For this review, take the finished solid that the model builds, in its own axes (mm). A direction names the side the tool comes from. Round coordinates to 2 decimals unless told otherwise and drop trailing zeros. Write each loop counter-clockwise with the first axis right and the second up, starting at its lowest first coordinate (ties: lowest second). Pieces come first, ordered by that corner, then holes.
from build123d import *

# Parameters (mm, degrees)
F0_R     = 12.5
F1_DEPTH = 3
F2_R     = 1
F3_DEPTH = 12.5
F4_R     = 2
F4_R_2   = 1
F5_DEPTH = 4
F7_DEPTH = 2


with BuildPart() as f1:
    # F0 (on Top) → F1 (new body, symmetric)
    with BuildSketch(Plane.XY):
        Circle(F0_R)
    extrude(amount=F1_DEPTH, both=True)

    # F2 (on Top) → F3 (cut, symmetric)
    with BuildSketch(Plane.XY):
        with Locations((0, -8)):
            Circle(F2_R)
        with Locations((-5.6568542495, -5.6568542495)):
            Circle(F2_R)
        with Locations((-8, 0)):
            Circle(F2_R)
        with Locations((-5.6568542495, 5.6568542495)):
            Circle(F2_R)
        with Locations((0, 8)):
            Circle(F2_R)
        with Locations((5.6568542495, 5.6568542495)):
            Circle(F2_R)
        with Locations((8, 0)):
            Circle(F2_R)
        with Locations((5.6568542495, -5.6568542495)):
            Circle(F2_R)
    extrude(amount=F3_DEPTH, both=True, mode=Mode.SUBTRACT)

    # F4 (on face) → F5 (cut)
    with BuildSketch(Plane.XY.offset(3)):
        with Locations((-5.6568542495, 5.6568542495)):
            Circle(F4_R)
        with Locations((-5.6568542495, 5.6568542495)):
            Circle(F4_R_2, mode=Mode.SUBTRACT)
        with Locations((-8, 0)):
            Circle(F4_R)
        with Locations((-8, 0)):
            Circle(F4_R_2, mode=Mode.SUBTRACT)
        with Locations((0, 8)):
            Circle(F4_R)
        with Locations((0, 8)):
            Circle(F4_R_2, mode=Mode.SUBTRACT)
        with Locations((8, 0)):
            Circle(F4_R)
        with Locations((8, 0)):
            Circle(F4_R_2, mode=Mode.SUBTRACT)
        with Locations((5.6568542495, 5.6568542495)):
            Circle(F4_R)
        with Locations((5.6568542495, 5.6568542495)):
            Circle(F4_R_2, mode=Mode.SUBTRACT)
        with Locations((5.6568542495, -5.6568542495)):
            Circle(F4_R)
        with Locations((5.6568542495, -5.6568542495)):
            Circle(F4_R_2, mode=Mode.SUBTRACT)
        with Locations((0, -8)):
            Circle(F4_R)
        with Locations((0, -8)):
            Circle(F4_R_2, mode=Mode.SUBTRACT)
        with Locations((-5.6568542495, -5.6568542495)):
            Circle(F4_R)
        with Locations((-5.6568542495, -5.6568542495)):
            Circle(F4_R_2, mode=Mode.SUBTRACT)
    extrude(amount=-F5_DEPTH, mode=Mode.SUBTRACT)

    # F6 (on face) → F7 (join)
    with BuildSketch(Plane.XY.offset(3)):
        Polygon((-0.2840909091, 1.25), (-1.25, 5.5), (-1.25, 1.25), align=None)
        Polygon((1.25, 5.5), (-1.25, 5.5), (-0.2840909091, 1.25), (1.25, 1.25), align=None)
        Polygon((-0.2840909091, 1.25), (-1.25, 1.25), (-1.25, -0.2840909091), (0, 0), align=None)
        Polygon((-1.25, -0.2840909091), (-1.25, 1.25), (-5.5, 1.25), (-5.5, -1.25), align=None)
        Polygon((1.25, 1.25), (-0.2840909091, 1.25), (0, 0), (1.25, 0.2840909091), align=None)
        Polygon((5.5, 1.25), (1.25, 1.25), (1.25, 0.2840909091), align=None)
        Polygon((0, 0), (-1.25, -0.2840909091), (-1.25, -1.25), (0.2840909091, -1.25), align=None)
        Polygon((-1.25, -1.25), (-1.25, -0.2840909091), (-5.5, -1.25), align=None)
        Polygon((1.25, 0.2840909091), (0, 0), (0.2840909091, -1.25), (1.25, -1.25), align=None)
        Polygon((5.5, 1.25), (1.25, 0.2840909091), (1.25, -1.25), (5.5, -1.25), align=None)
        Polygon((0.2840909091, -1.25), (-1.25, -1.25), (-1.25, -5.5), (1.25, -5.5), align=None)
        Polygon((1.25, -1.25), (0.2840909091, -1.25), (1.25, -5.5), align=None)
    extrude(amount=F7_DEPTH)


solid = f1.part
(1) Mouldability with a two-part tool opening along Y and no side actions: class faces 6 (the face through (1.25, -3, 4)), 7 (the face through (0, 5.5, 4)), 8 (the face through (6.5, -6.5, -1)) as pulls with the +Y half, pulls with the -Y half, needs draft (parallel to the pull), parting line crosses it, or undercut.
Geometry check:
face 6: needs draft
face 7: pulls with the +Y half
face 8: undercut
(2) We need section C-C, the plane z = 1.25. State how many separate pieces and enclosed holes the cut face has, and give its area (3 significant figures).
Geometry check:
separate pieces: 1
enclosed holes: 8
area: 390 mm2
(3) For line 1 along Y through (x, z) = (0, -2.05); line 2 along Y through (x, z) = (4.25, -0.5); line 3 along Z through (x, y) = (-5.5, -7.75), list the stretches that pass through material, from the lowest coordinate up.
Geometry check:
line 1: y = -12.5 to -9, -7 to 7, 9 to 12.5
line 2: y = -11.76 to -7.08, -4.24 to 4.24, 7.08 to 11.76
line 3: z = -3 to 3
(4) We need section A-A, the plane y = 0. Give the boundary of the cut face in (x, z).
Geometry check:
outline: (-12.5, -3) - (-9, -3) - (-9, -1) - (-10, -1) - (-10, 3) - (-12.5, 3) - close; (-7, -3) - (7, -3) - (7, -1) - (6, -1) - (6, 3) - (5.5, 3) - (5.5, 5) - (-5.5, 5) - (-5.5, 3) - (-6, 3) - (-6, -1) - (-7, -1) - close; (9, -3) - (12.5, -3) - (12.5, 3) - (10, 3) - (10, -1) - (9, -1) - close
(5) We need section D-D, the plane y = 8. Give the boundary of the cut face in (x, z).
Geometry check:
outline: (-9.6, -3) - (-1, -3) - (-1, -1) - (-2, -1) - (-2, 3) - (-9.6, 3) - close; (1, -3) - (9.6, -3) - (9.6, 3) - (2, 3) - (2, -1) - (1, -1) - close
(6) For pin 1 Ø1.6 at (y, z) = (-3.5, 3.5) entering from +X; pin 2 Ø1.6 at (y, z) = (4, 4) entering from +X; pin 3 Ø1.5 at (y, z) = (-1, 3) entering from -X; pin 4 Ø1.8 at (x, y) = (5.66, 5.66) entering from -Z (3 decimals), all flat-tipped, find the tip position at first contact; note any pin that passes through.
Geometry check:
pin 1: stops at x = 12.16
pin 2: stops at x = 1.25
pin 3: stops at x = -12.5
pin 4: passes through
(7) For faces 1 (the face through (0, 0, 5)), 2 (the face through (-3, 1.25, 4)), 3 (the face through (-1.25, -3, 4)), 4 (the face through (-7, 5, -1)), 5 (the face through (6.12, 4.77, -1.99)), list the 3-axis set-ups (+Z, -Z, +X, -X, +Y, -Y) from which the entire face can be reached by the end or side of a thin tool; tool diameter is ignored.
Geometry check:
face 1: +Z, +X, -X, +Y, -Y
face 2: +Z, -X, +Y
face 3: +Z, -X, -Y
face 4: +Z
face 5: +Z, -Z
